```python
from build123d import *

# Parameters (mm, degrees)
IZIM1_R                     = 3.25
Y_KSEKLIK_EKSTR_ZYON1_DEPTH = 6.5


with BuildPart() as part:
    # Çizim1 → Yükseklik-Ekstrüzyon1 (new body)
    with BuildSketch(Plane.XY):
        Polygon((7.505553499, 0), (3.75277675, 6.5), (-3.75277675, 6.5), (-7.505553499, 0), (-3.75277675, -6.5), (3.75277675, -6.5), align=None)
        with Locations(Location((0, 0, 0), (0, 0, 180))):
            Circle(IZIM1_R, mode=Mode.SUBTRACT)
    extrude(amount=Y_KSEKLIK_EKSTR_ZYON1_DEPTH)

    # Çizim2 → Kes-Döndür1 (revolve, cut)
    with BuildSketch(Plane(origin=(0, 0, 0), x_dir=(1, 0, 0), z_dir=(0, 1, 0))):
        Polygon((-7.505553499, 0), (-6.505553499, 0), (-7.505553499, -0.5), align=None)
        Polygon((-7.505553499, -6.5), (-7.505553499, -6), (-6.505553499, -6.5), align=None)
    revolve(axis=Axis((0, 0, 0), (0, 0, 1)), mode=Mode.SUBTRACT)


solid = part.part
```
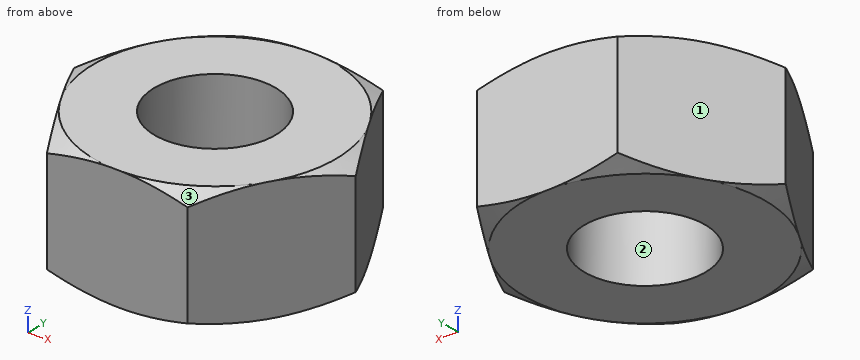
The listing builds one solid part. Answer for the finished solid, in the listing's coordinates (mm). Face numbers are marked on the shaded views. Round coordinates to 2 decimals unless told otherwise and drop trailing zeros. Loops run counter-clockwise (first coordinate to the right, second up) from the corner with the lowest first, then second, coordinate; pieces in that order, holes last.
Q1. Section A-A, the plane x = 0 is taken. Determine the outline of the cut face in (y, z), then the cut area to 4 significant figures.
Q2. Section B-B, the plane z = 3.25 is taken. Determine the outline of the cut face in (x, y), then the cut area to 3 significant figures.
Q3. For a pull along Y with two mould halves and no side action, classify the marked faces 1, 2 and 3 as released by +Y, released by -Y, zero draft, split by the parting line, or undercut.
Q4. Given pin 1 Ø1.5 at (y, z) = (2, 2) entering from +X; pin 2 Ø1.5 at (x, y) = (-5.5, 3.5) entering from -Z; pin 3 Ø2 at (y, z) = (-3, 2) entering from -X; pin 4 Ø1.5 at (y, z) = (3, 0.5) entering from -X, each flat-ended and moving along its own axis, determine where each tip first touches the part or whether it passes through.
Q5. Find the intervals of material crossed by line 1 (Y direction, x = 0, z = 2.25); line 2 (X direction, y = -0.75, z = 4.25); line 3 (X direction, y = -1.5, z = 6.25), in increasing order.
Completed:
1. outline: (-6.5, 0) - (-3.25, 0) - (-3.25, 6.5) - (-6.5, 6.5) - close; (3.25, 0) - (6.5, 0) - (6.5, 6.5) - (3.25, 6.5) - close
1. area: 42.25 mm2
2. outline: (-7.51, 0) - (-3.75, -6.5) - (3.75, -6.5) - (7.51, 0) - (3.75, 6.5) - (-3.75, 6.5) - close; hole circle Ø6.5 at (0, 0)
2. area: 113 mm2
3. face 1: released by +Y
3. face 2: undercut
3. face 3: released by -Y
4. pin 1: stops at x = 6.78
4. pin 2: stops at z = 0
4. pin 3: stops at x = -6.35
4. pin 4: stops at x = -6.21
5. line 1: y = -6.5 to -3.25, 3.25 to 6.5
5. line 2: x = -7.07 to -3.16, 3.16 to 7.07
5. line 3: x = -6.64 to -2.88, 2.88 to 6.64
